from build123d import *

# Parameters (mm, degrees)
SKETCH1_R           = 34.5
SKETCH1_R_2         = 32.5
BOSS_EXTRUDE1_DEPTH = 512
CUT_EXTRUDE1_START  = -12
SKETCH3_R           = 33
SKETCH3_R_2         = 32.5
CUT_EXTRUDE1_DEPTH  = 12
CUT_EXTRUDE3_START  = -18
SKETCH4_R           = 34.5
SKETCH4_R_2         = 34.25
CUT_EXTRUDE3_DEPTH  = 18
SKETCH5_R           = 34.5
SKETCH5_R_2         = 34.25
CUT_EXTRUDE4_DEPTH  = 18


with BuildPart() as part:
    # Sketch1 → Boss-Extrude1 (new body)
    with BuildSketch(Plane.XY):
        Circle(SKETCH1_R)
        Circle(SKETCH1_R_2, mode=Mode.SUBTRACT)
    extrude(amount=BOSS_EXTRUDE1_DEPTH)

    # Sketch3 → Cut-Extrude1 (cut)
    with BuildSketch(Plane.XY.offset(512).offset(CUT_EXTRUDE1_START)):
        Circle(SKETCH3_R)
        Circle(SKETCH3_R_2, mode=Mode.SUBTRACT)
    extrude(amount=CUT_EXTRUDE1_DEPTH, mode=Mode.SUBTRACT)

    # Sketch4 → Cut-Extrude3 (cut)
    with BuildSketch(Plane.XY.offset(512).offset(CUT_EXTRUDE3_START)):
        Circle(SKETCH4_R)
        Circle(SKETCH4_R_2, mode=Mode.SUBTRACT)
    extrude(amount=CUT_EXTRUDE3_DEPTH, mode=Mode.SUBTRACT)

    # Sketch5 → Cut-Extrude4 (cut)
    with BuildSketch(Plane(origin=(0, 0, 0), x_dir=(-1, 0, 0), z_dir=(0, 0, -1))):
        Circle(SKETCH5_R)
        with Locations(Location((0, 0, 0), (0, 0, 180))):
            Circle(SKETCH5_R_2, mode=Mode.SUBTRACT)
    extrude(amount=-CUT_EXTRUDE4_DEPTH, mode=Mode.SUBTRACT)


solid = part.part
Check sheet for the modelled part. Datum: model origin and axes. Units: mm. A direction names the side the tool comes from. Round coordinates to 2 decimals unless told otherwise and drop trailing zeros. Order: outer loops, then holes, each group sorted by start corner. A loop starts at its lowest first (then second) coordinate and runs counter-clockwise, first axis right, second up.
Q1. Cross-section at C-C, the plane z = 126. Enter the section's corners in (x, y).
Filled sheet:
outline: circle Ø69 at (0, 0); hole circle Ø65 at (0, 0)
Q2. Depth check by flat-ended pin: P1, Ø20.5, axis at x = -13, y = -13.5, coming from the -Z side; P2, Ø1, axis at x = -4.5, z = 365, coming from the -Y side; P3, Ø5, axis at y = 20, z = 63, coming from the -X side; P4, Ø8, axis at y = 11, z = 292, coming from the +X side. Enter the tip coordinate at first touch or a pass-through.
Filled sheet:
P1: passes through
P2: stops at y = -34.27
P3: stops at x = -29.73
P4: stops at x = 33.78
Q3. Set-up check for faces 1 (the face through (31, 9.76, 246.5)), 2 (the face through (24.29, -21.85, 500)): record each of +Z, -Z, +X, -X, +Y, -Y from which the full face is reachable in a straight line by a thin tool's end or side.
Filled sheet:
face 1: +Z, -Z
face 2: +Z
Q4. Cross-section at A-A, the plane y = 0. Enter the section's corners in (x, z).
Filled sheet:
outline: (-34.5, 18) - (-34.25, 18) - (-34.25, 0) - (-32.5, 0) - (-32.5, 500) - (-33, 500) - (-33, 512) - (-34.25, 512) - (-34.25, 494) - (-34.5, 494) - close; (32.5, 0) - (34.25, 0) - (34.25, 18) - (34.5, 18) - (34.5, 494) - (34.25, 494) - (34.25, 512) - (33, 512) - (33, 500) - (32.5, 500) - close
Q5. Scan lines: L1, parallel to Y at x = 0, z = 192; L2, parallel to Y at x = 0, z = 506.5; L3, parallel to X at y = -2.5, z = 113. Record each from-to range of solid material in increasing order.
Filled sheet:
L1: y = -34.5 to -32.5, 32.5 to 34.5
L2: y = -34.25 to -33, 33 to 34.25
L3: x = -34.41 to -32.4, 32.4 to 34.41
Q6. Cross-section at B-B, the plane x = 27. Enter the section's corners in (y, z).
Filled sheet:
outline: (-21.48, 18) - (-21.07, 18) - (-21.07, 0) - (-18.09, 0) - (-18.09, 500) - (-18.97, 500) - (-18.97, 512) - (-21.07, 512) - (-21.07, 494) - (-21.48, 494) - close; (18.09, 0) - (21.07, 0) - (21.07, 18) - (21.48, 18) - (21.48, 494) - (21.07, 494) - (21.07, 512) - (18.97, 512) - (18.97, 500) - (18.09, 500) - close
Q7. Draft check along Y on faces 3 (the face through (32.907, 10.363, 252.668)), 4 (the face through (30.5, -12.6, 505.9)), 5 (the face through (20, 26, 0)). Enter one of: pulls with the +Y half, pulls with the -Y half, needs draft (parallel to the pull), parting line crosses it, or undercut.
Filled sheet:
face 3: parting line crosses it
face 4: undercut
face 5: needs draft
